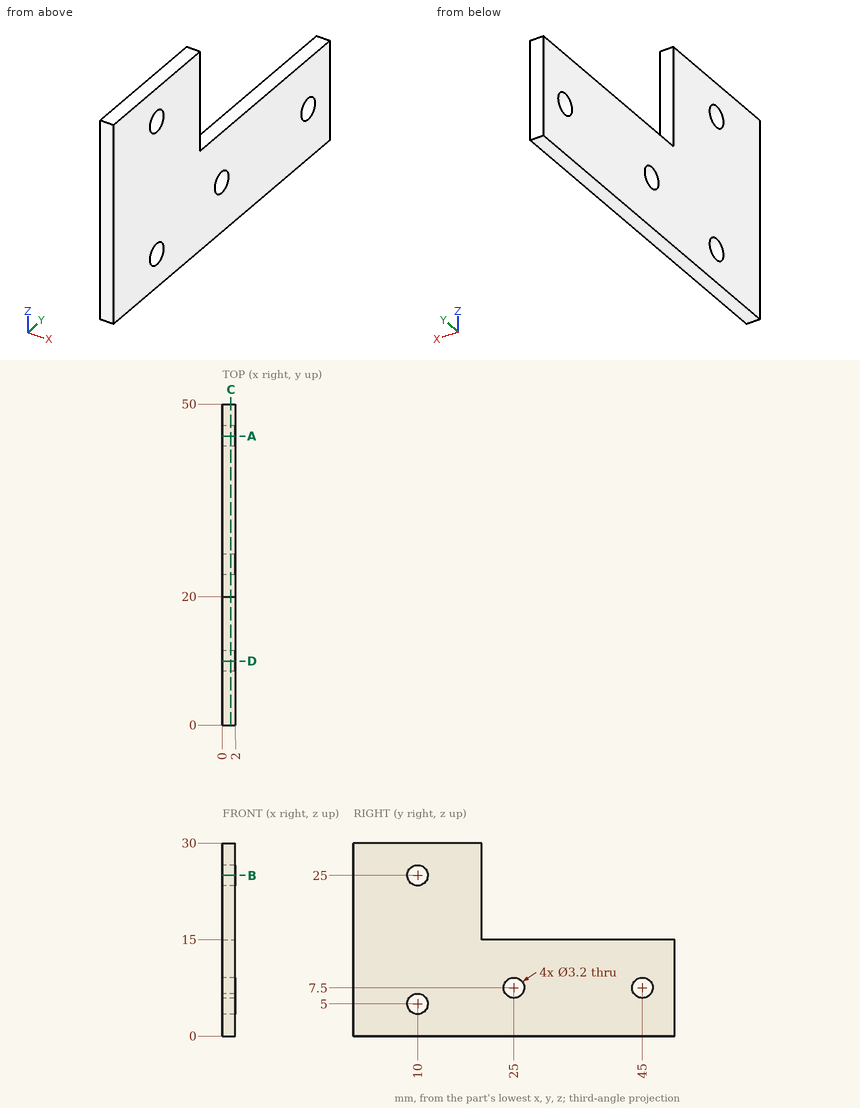
Input: dimensioned drawing with shaded views. Units: mm. Origin: part minimum x, y, z. Coordinates: 2 decimals unless noted, no trailing zeros. Loops run counter-clockwise (first coordinate to the right, second up) from the corner with the lowest first, then second, coordinate; pieces in that order, holes last. Notation, with made-up numbers: (54.5, 62.25) -> (62.5, 62.25) arc R16 cw to (62.5, 79.25) -> close; hole circle Ø7 at (-25, 7). An arc over 180 degrees is marked (long way). Use a Markdown table: item, result. Add a question column.
(1) Line query: line 1 along Z through (x, y) = (0.6, 10); line 2 along Y through (x, z) = (1.3, 7.5); line 3 along Y through (x, z) = (0.75, 25). Output: solid intervals per line, ascending.
(2) Section query C-C, the plane x = 1.3. Return loops of the section in (y, z).
(3) Section query A-A, the plane y = 45. Return loops of the section in (x, z), plus the area to 3 significant figures.
(4) Pin query (flat end, axial travel): pin 1 Ø0.6 at (x, z) = (1.5, 23) entering from +Y; pin 2 Ø1 at (x, y) = (1, 31.5) entering from +Z. Return the tip coordinate at first contact, or that it passes through.
(5) Section query D-D, the plane y = 10. Return loops of the section in (x, z), plus the area to 3 significant figures.
(6) Section query B-B, the plane z = 25. Return loops of the section in (x, y).
Answer:
| question | item | result |
|---|---|---|
| 1 | line 1 | z = 0 to 3.4, 6.6 to 23.4, 26.6 to 30 |
| 1 | line 2 | y = 0 to 23.4, 26.6 to 43.4, 46.6 to 50 |
| 1 | line 3 | y = 0 to 8.4, 11.6 to 20 |
| 2 | outline | (0, 0) -> (50, 0) -> (50, 15) -> (20, 15) -> (20, 30) -> (0, 30) -> close; hole circle Ø3.2 at (10, 5); hole circle Ø3.2 at (10, 25); hole circle Ø3.2 at (25, 7.5); hole circle Ø3.2 at (45, 7.5) |
| 3 | outline | (0, 0) -> (2, 0) -> (2, 5.9) -> (0, 5.9) -> close; (0, 9.1) -> (2, 9.1) -> (2, 15) -> (0, 15) -> close |
| 3 | area | 23.6 mm^2 |
| 4 | pin 1 | stops at y = 20 |
| 4 | pin 2 | stops at z = 15 |
| 5 | outline | (0, 0) -> (2, 0) -> (2, 3.4) -> (0, 3.4) -> close; (0, 6.6) -> (2, 6.6) -> (2, 23.4) -> (0, 23.4) -> close; (0, 26.6) -> (2, 26.6) -> (2, 30) -> (0, 30) -> close |
| 5 | area | 47.2 mm^2 |
| 6 | outline | (0, 0) -> (2, 0) -> (2, 8.4) -> (0, 8.4) -> close; (0, 11.6) -> (2, 11.6) -> (2, 20) -> (0, 20) -> close |
